Read the model definition and answer for the solid it produces. Units are mm, in the model's axes. Coordinates: 2 decimals unless noted, no trailing zeros. Loops run counter-clockwise (first coordinate to the right, second up) from the corner with the lowest first, then second, coordinate; pieces in that order, holes last. Notation, with made-up numbers: M -6.75,56 L 45.25,56 A17 cw 45.25,87 Z; hole C 86,48.5 d6. An arc over 180 degrees is marked long. One line per item, written item: value. Start each with the question number.
1. Consider probe 1 along Y at (x, z) = (0, 310.25); probe 2 along Z at (x, y) = (-0.5, -1.25); probe 3 along X at (y, z) = (-2.75, 115). Determine where each line is inside the solid, lowest interval first.
2. The part is cut by section C-C (z = 246). Write down the section's boundary in (x, y).
3. The part is cut by section A-A (x = 0). Write down the section's boundary in (y, z), then the cut area to 3 significant figures.
4. Flat-ended cylindrical pins translate along their axes: pin 1 (5 mm diameter, centred on y = -4, z = 184.5, fed in from +X); pin 2 (2.5 mm diameter, centred on x = 0, y = 0, fed in from -Z); pin 3 (5.5 mm diameter, centred on x = 0, y = 0, fed in from -Z); pin 4 (5 mm diameter, centred on y = -3.5, z = 245.5, fed in from +X). Find the tip coordinate at first contact, or state that the pin passes through.
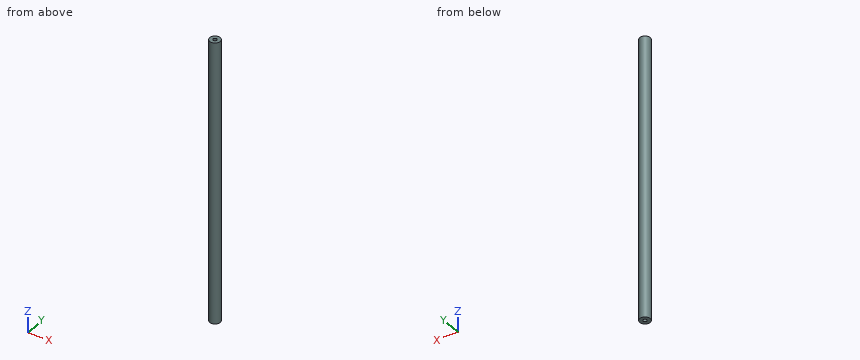
```python
from build123d import *

# Parameters (mm, degrees)
SKETCH1_R           = 6
BOSS_EXTRUDE1_DEPTH = 320
SKETCH2_R           = 2.15
CUT_EXTRUDE1_DEPTH  = 20
SKETCH3_R           = 2.15
CUT_EXTRUDE2_DEPTH  = 20


with BuildPart() as part:
    # Sketch1 → Boss-Extrude1 (new body)
    with BuildSketch(Plane.XY):
        Circle(SKETCH1_R)
    extrude(amount=BOSS_EXTRUDE1_DEPTH)

    # Sketch2 → Cut-Extrude1 (cut)
    with BuildSketch(Plane.XY.offset(320)):
        Circle(SKETCH2_R)
    extrude(amount=-CUT_EXTRUDE1_DEPTH, mode=Mode.SUBTRACT)

    # Sketch3 → Cut-Extrude2 (cut)
    with BuildSketch(Plane(origin=(0, 0, 0), x_dir=(-1, 0, 0), z_dir=(0, 0, -1))):
        Circle(SKETCH3_R)
    extrude(amount=-CUT_EXTRUDE2_DEPTH, mode=Mode.SUBTRACT)


solid = part.part
```
Answer block:
1. probe 1: y = -6 to -2.15, 2.15 to 6
1. probe 2: z = 20 to 300
1. probe 3: x = -5.33 to 5.33
2. outline: C 0,0 d12
3. outline: M -6,0 L -2.15,0 L -2.15,20 L 2.15,20 L 2.15,0 L 6,0 L 6,320 L 2.15,320 L 2.15,300 L -2.15,300 L -2.15,320 L -6,320 Z
3. area: 3,670 mm2
4. pin 1: stops at x = 5.81
4. pin 2: stops at z = 20
4. pin 3: stops at z = 0
4. pin 4: stops at x = 5.92
